from build123d import *

# Parameters (mm, degrees)
SKICA1_R                 = 23.5
P_IDAT_VYSUNUT_M1_DEPTH  = 3
SKICA2_R                 = 5.65
ODEBRAT_VYSUNUT_M1_DEPTH = 3
SKICA3_W                 = 4.15
SKICA3_H                 = 3
SKICA3_W_2               = 3
SKICA3_H_2               = 4.15
ODEBRAT_VYSUNUT_M2_DEPTH = 3


with BuildPart() as part:
    # Skica1 → Přidat vysunutím1 (new body)
    with BuildSketch(Plane(origin=(0, 0, 0), x_dir=(1, 0, 0), z_dir=(0, 1, 0))):
        with Locations(Location((0, 0, 0), (0, 0, 270))):
            Circle(SKICA1_R)
    extrude(amount=P_IDAT_VYSUNUT_M1_DEPTH)

    # Skica2 → Odebrat vysunutím1 (cut)
    with BuildSketch(Plane(origin=(0, 3, 0), x_dir=(1, 0, 0), z_dir=(0, 1, 0))):
        with Locations(Location((0, 0, 0), (0, 0, 270))):
            Circle(SKICA2_R)
    extrude(amount=-ODEBRAT_VYSUNUT_M1_DEPTH, mode=Mode.SUBTRACT)

    # Skica3 → Odebrat vysunutím2 (cut)
    with BuildSketch(Plane.XZ):
        with Locations((20.075, 0)):
            Rectangle(SKICA3_W, SKICA3_H)
        with Locations((0, 20.075)):
            Rectangle(SKICA3_W_2, SKICA3_H_2)
        with Locations((0, -20.075)):
            Rectangle(SKICA3_W_2, SKICA3_H_2)
        with Locations((-20.075, 0)):
            Rectangle(SKICA3_W, SKICA3_H)
    extrude(amount=-ODEBRAT_VYSUNUT_M2_DEPTH, mode=Mode.SUBTRACT)


solid = part.part
Design review of the part built by this model. Coordinates are the model's own, in mm. A direction names the side the tool comes from. Round coordinates to 2 decimals unless told otherwise and drop trailing zeros. Write each loop counter-clockwise with the first axis right and the second up, starting at its lowest first coordinate (ties: lowest second). Pieces come first, ordered by that corner, then holes. Notation, with made-up numbers: (57.25, 46) - (85.25, 46) arc R17 ccw to (85.25, 69) - close; hole circle Ø11 at (57.25, 24.25). An arc over 180 degrees is marked (long way). Use a Markdown table: item, result. Add a question column.
1. We need section C-C (x = 0). State the section outline as (y, z) points, then the cut area to 3 significant figures.
2. Wall thickness on probe 1 along X at (y, z) = (2.3, 0); probe 2 along Z at (x, y) = (-19, 1.2); probe 3 along X at (y, z) = (2.25, 21): over which ranges is each line inside the solid? List them lowest first.
3. We need section A-A (z = 0). State the section outline as (x, y) points, then the cut area to 3 significant figures.
4. Mouldability with a two-part tool opening along Z and no side actions: class faces 3 (the face through (22.15, 1, 0)), 4 (the face through (-5, 3, 5)), 5 (the face through (15.88, 1.48, -17.32)) as +Z half, -Z half, draft (parallel to the pull), parting line (faces both ways), or undercut.
5. We need section B-B (y = 1.1). State the section outline as (x, z) points.
6. For faces 1 (the face through (20, 1, -1.5)), 2 (the face through (-5, 0, 5)), list the 3-axis set-ups (+Z, -Z, +X, -X, +Y, -Y) from which the entire face can be reached by the end or side of a thin tool; tool diameter is ignored.
7. We need section D-D (x = -20). State the section outline as (y, z) points, then the cut area to 3 significant figures.
8. Clearance check with flat-ended pins moving along their axes: pin 1 (1.5 mm diameter, centred on y = 2, z = -20, fed in from +X); pin 2 (1.5 mm diameter, centred on y = 1.5, z = 0.5, fed in from -X); pin 3 (1.5 mm diameter, centred on x = -19.5, y = 2, fed in from -Z). State where each tip first meets the part, or that it passes through.
Output:
| question | item | result |
|---|---|---|
| 1 | outline | (0, -23.5) - (3, -23.5) - (3, -22.15) - (0, -22.15) - close; (0, -18) - (3, -18) - (3, -5.65) - (0, -5.65) - close; (0, 5.65) - (3, 5.65) - (3, 18) - (0, 18) - close; (0, 22.15) - (3, 22.15) - (3, 23.5) - (0, 23.5) - close |
| 1 | area | 82.2 mm2 |
| 2 | probe 1 | x = -23.5 to -22.15, -18 to -5.65, 5.65 to 18, 22.15 to 23.5 |
| 2 | probe 2 | z = -13.83 to -1.5, 1.5 to 13.83 |
| 2 | probe 3 | x = -10.55 to -1.5, 1.5 to 10.55 |
| 3 | outline | (-23.5, 0) - (-22.15, 0) - (-22.15, 3) - (-23.5, 3) - close; (-18, 0) - (-5.65, 0) - (-5.65, 3) - (-18, 3) - close; (5.65, 0) - (18, 0) - (18, 3) - (5.65, 3) - close; (22.15, 0) - (23.5, 0) - (23.5, 3) - (22.15, 3) - close |
| 3 | area | 82.2 mm2 |
| 4 | face 3 | undercut |
| 4 | face 4 | draft |
| 4 | face 5 | parting line |
| 5 | outline | circle Ø47 at (0, 0); hole (-22.15, -1.5) - (-18, -1.5) - (-18, 1.5) - (-22.15, 1.5) - close; hole circle Ø11.3 at (0, 0); hole (-1.5, -22.15) - (1.5, -22.15) - (1.5, -18) - (-1.5, -18) - close; hole (-1.5, 18) - (1.5, 18) - (1.5, 22.15) - (-1.5, 22.15) - close; hole (18, -1.5) - (22.15, -1.5) - (22.15, 1.5) - (18, 1.5) - close |
| 6 | face 1 | +Y, -Y |
| 6 | face 2 | +Z, -Z, +X, -X, -Y |
| 7 | outline | (0, -12.34) - (3, -12.34) - (3, -1.5) - (0, -1.5) - close; (0, 1.5) - (3, 1.5) - (3, 12.34) - (0, 12.34) - close |
| 7 | area | 65.0 mm2 |
| 8 | pin 1 | stops at x = 13.48 |
| 8 | pin 2 | stops at x = -23.5 |
| 8 | pin 3 | stops at z = -14.17 |
